Job drawing, mm, ordinate dimensions from the low corner. One solid piece. A direction names the side the tool comes from. Coordinates: 2 decimals unless noted, no trailing zeros. Write each loop counter-clockwise with the first axis right and the second up, starting at its lowest first coordinate (ties: lowest second). Pieces come first, ordered by that corner, then holes. Notation, with made-up numbers: (-15.5, 52.25) - (43.5, 52.25) arc R18 cw to (43.5, 73.25) - close; hole circle Ø4 at (73.5, 48.5). An arc over 180 degrees is marked (long way). Use one line per item in the form item = value. Start each with the question number.
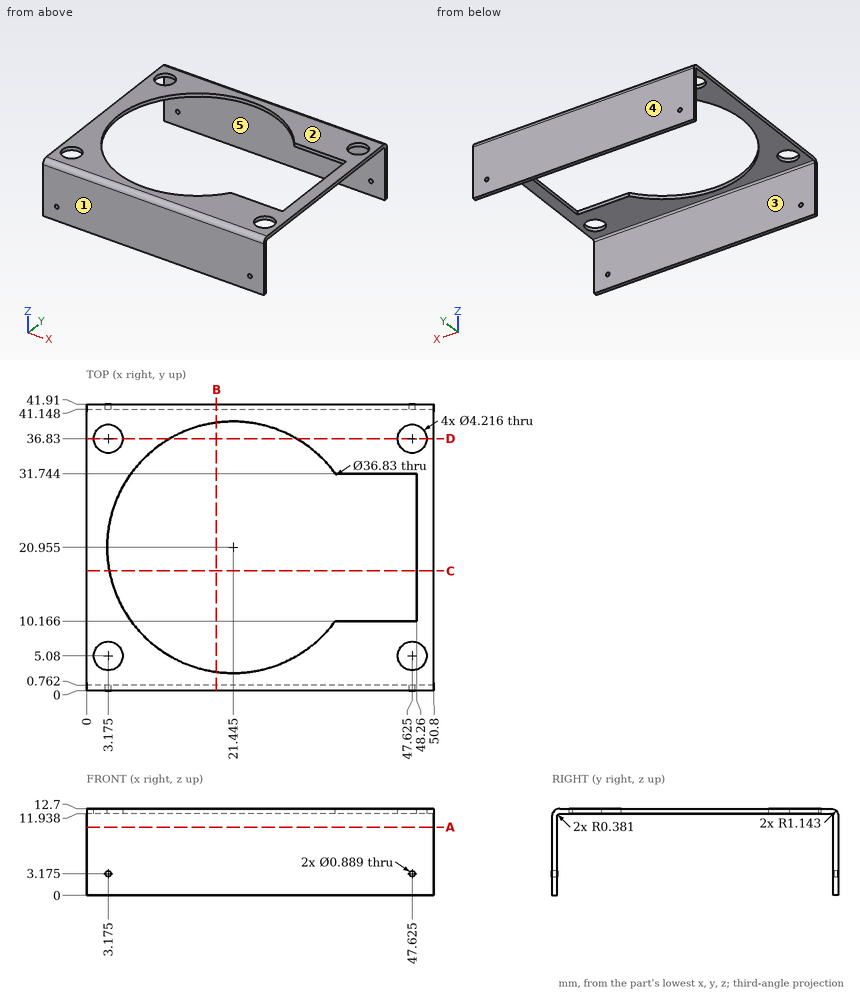
Q1. Slice it at B-B (x = 19). List the corners of the cut face in (y, z).
Q2. Slice it at A-A (z = 10). List the corners of the cut face in (x, y).
Q3. Which spindle directions (+Z, -Z, +X, -X, +Y, -Y) get a long thin tool onto all of the face, cutting with end or side? Do the marked faces 4 and 5. Say none if no direction does.
Q4. Drill centre lines: probe 1 along Y at (x, z) = (38, 4.75); probe 2 along X at (y, z) = (6, 12.25); probe 3 along Z at (x, y) = (37, 6.5). Where is each one in solid material? Low to high.
Q5. Mould opens along Y. For the marked faces 1, 2 and 3 say: released by +Y, released by -Y, zero draft, split by the parting line, or undercut.
Q6. Slice it at C-C (y = 17.5). List the corners of the cut face in (x, z).
Q7. Pin check, flat tips, straight feed: P1, Ø5.5, axis at x = 3.175, y = 5.08, coming from the +Z side; P2, Ø0.6, axis at x = 44.5, z = 12.5, coming from the +Y side; P3, Ø5, axis at x = 3.175, y = 36.83, coming from the -Z side. Stop position of each tip, or through.
Q8. Slice it at D-D (y = 36.83). List the corners of the cut face in (x, z).
Solution:
q1.outline = (0, 0) - (0.76, 0) - (0.76, 11.56) arc R0.38 cw to (1.14, 11.94) - (2.7, 11.94) - (2.7, 12.7) - (1.14, 12.7) arc R1.14 ccw to (0, 11.56) - close; (39.21, 11.94) - (40.77, 11.94) arc R0.38 cw to (41.15, 11.56) - (41.15, 0) - (41.91, 0) - (41.91, 11.56) arc R1.14 ccw to (40.77, 12.7) - (39.21, 12.7) - close
q2.outline = (0, 0) - (50.8, 0) - (50.8, 0.76) - (0, 0.76) - close; (0, 41.15) - (50.8, 41.15) - (50.8, 41.91) - (0, 41.91) - close
q3.face_4 = +Z, -Z, +X, -X, +Y
q3.face_5 = -Z, +X, -X
q4.probe_1 = 0 to 0.76, 41.15 to 41.91
q4.probe_2 = 0 to 1.28, 5.07 to 10.7, 32.19 to 45.73, 49.52 to 50.8
q4.probe_3 = 11.94 to 12.7
q5.face_1 = released by -Y
q5.face_2 = zero draft
q5.face_3 = undercut
q6.outline = (0, 11.94) - (3.36, 11.94) - (3.36, 12.7) - (0, 12.7) - close; (48.26, 11.94) - (50.8, 11.94) - (50.8, 12.7) - (48.26, 12.7) - close
q7.P1 = 12.7
q7.P2 = 41.71
q7.P3 = 11.94
q8.outline = (0, 11.94) - (1.07, 11.94) - (1.07, 12.7) - (0, 12.7) - close; (5.28, 11.94) - (12.11, 11.94) - (12.11, 12.7) - (5.28, 12.7) - close; (30.78, 11.94) - (45.52, 11.94) - (45.52, 12.7) - (30.78, 12.7) - close; (49.73, 11.94) - (50.8, 11.94) - (50.8, 12.7) - (49.73, 12.7) - close
